Build history of the part. All positions in model axes, mm. A direction names the side the tool comes from. Give positions to 0.01 mm unless a question says otherwise; leave off trailing zeros. Loops run counter-clockwise (first coordinate to the right, second up) from the corner with the lowest first, then second, coordinate; pieces in that order, holes last. Notation, with made-up numbers: (-32, -4) -> (-8, -4) arc R21 ccw to (-8, 18) -> close; hole circle Ø5 at (37.25, 39.5). An arc over 180 degrees is marked (long way). Answer as a JSON object with one key per item and string values. Group by question number.
Q1. Band-saw the part on A-A, the plane z = 1.15. Count the separate pieces of the cut face and the enclosed holes in it, plus the area to 3 significant figures.
Q2. Band-saw the part on B-B, the plane y = 80. Write the cut outline in (x, z).
Q3. Drop flat-ended pins along their axis: pin 1 (2 mm diameter, centred on x = 57.75, y = -19.5, fed in from +Z); pin 2 (1.5 mm diameter, centred on x = -70, z = 2, fed in from +Y); pin 3 (2.5 mm diameter, centred on y = -83, z = 3.5, fed in from +X); pin 4 (1.5 mm diameter, centred on y = 4.5, z = 3, fed in from -X). Give the stop position or say it passes through.
Q4. Tool access for faces 1 (the flat face through (-72, -75, 3)), 2 (the flat face through (67, -86, 3)), 3 (the flat face through (67, 86, 3)): list every direction of +Z, -Z, +X, -X, +Y, -Y with a clear straight run to the whole face (end or side of a thin tool).
Q5. Two-plate mould, pull along X, no slides. Class faces 4 (the flat face through (1, 55.3, 2)), 5 (the flat face through (37.65, 72, 2)), 6 (the flat face through (-67, 86, 3)), 7 (the flat face through (72, -75, 3)): pulls with the +X half, pulls with the -X half, needs draft (parallel to the pull), parting line crosses it, or undercut.
Q6. Wall check: probe 1 along X at (y, z) = (45.3, 1.6); probe 2 along X at (y, z) = (-80.5, 3.25); probe 3 along Y at (x, z) = (-58.05, 1.2). Give the ranges that are in metal, low to high. Write a range as from..to.
from build123d import *

# Parameters (mm, degrees)
PAD002_DEPTH    = 5
SKETCH002_R     = 0.9
SKETCH002_R_2   = 1.4
POCKET002_DEPTH = 5
SKETCH009_W     = 134
SKETCH009_H     = 6
POCKET009_DEPTH = 2


with BuildPart() as part:
    # Sketch004 → Pad002 (new body)
    with BuildSketch(Plane(origin=(0, 0, 5), x_dir=(1, 0, 0), z_dir=(0, 0, -1))):
        Polygon((-67, 97.5), (67, 97.5), (67, 75), (77, 75), (77, 25), (67, 25), (67, 0), (67, -25), (77, -25), (77, -75), (67, -75), (67, -97.5), (-67, -97.5), (-67, -75), (-77, -75), (-77, -25), (-67, -25), (-67, 0), (-67, 25), (-77, 25), (-77, 75), (-67, 75), align=None)
    extrude(amount=PAD002_DEPTH)

    # Sketch002 (on Face4 of Pad001) → Pocket002 (cut)
    with BuildSketch(Plane(origin=(0, 0, 0), x_dir=(1, 0, 0), z_dir=(0, 0, -1))):
        with Locations((-2, 80.5)):
            Circle(SKETCH002_R)
        with Locations((-60, 80.5)):
            Circle(SKETCH002_R)
        with Locations((-60, 31.5)):
            Circle(SKETCH002_R)
        with Locations((-2, 31.5)):
            Circle(SKETCH002_R)
        with Locations((-58.05, 19.5)):
            Circle(SKETCH002_R_2)
        with Locations((57.75, 19.5)):
            Circle(SKETCH002_R_2)
        with Locations((-58.05, -45.3)):
            Circle(SKETCH002_R_2)
        with Locations((57.75, -45.3)):
            Circle(SKETCH002_R_2)
        Polygon((37.65, -55.3), (37.65, -89.6), (-37.65, -89.6), (-37.65, -55.3), (0, -55.3), align=None)
    extrude(amount=-POCKET002_DEPTH, mode=Mode.SUBTRACT)

    # Sketch009 (on Face4 of Pocket002) → Pocket009 (cut)
    with BuildSketch(Plane.XY.offset(5)):
        with Locations((0, -90.5)):
            Rectangle(SKETCH009_W, SKETCH009_H)
    extrude(amount=-POCKET009_DEPTH, mode=Mode.SUBTRACT)


solid = part.part
Worked answers:
{
 "1": {"separate pieces": "1", "enclosed holes": "9", "area": "25,500 mm2"},
 "2": {"outline": "(-67, 0) -> (-37.65, 0) -> (-37.65, 5) -> (-67, 5) -> close; (37.65, 0) -> (67, 0) -> (67, 5) -> (37.65, 5) -> close"},
 "3": {"pin 1": "through", "pin 2": "y = 75", "pin 3": "x = 67", "pin 4": "x = -67"},
 "4": {"face 1": "+Z, -Z, -X, -Y", "face 2": "+Z, -Z, +X, -Y", "face 3": "+Z, -Z, +X, +Y"},
 "5": {"face 4": "undercut", "face 5": "undercut", "face 6": "pulls with the -X half", "face 7": "needs draft"},
 "6": {"probe 1": "-77..-59.45, -56.65..56.35, 59.15..77", "probe 2": "-67..-60.9, -59.1..-2.9, -1.1..67", "probe 3": "-97.5..-20.9, -18.1..43.9, 46.7..97.5"}
}
